Build history of the part. All positions in model axes, mm. A direction names the side the tool comes from. Coordinates: 2 decimals unless noted, no trailing zeros. Write each loop counter-clockwise with the first axis right and the second up, starting at its lowest first coordinate (ties: lowest second). Pieces come first, ordered by that corner, then holes.
```python
from build123d import *

# Parameters (mm, degrees)
SKETCH1_R          = 72.5
BASE_FLANGE1_DEPTH = 1


# Read off the part's stored shape, not the designer's step: Edge-Flange1
# Sheet-metal steps are written as plain solids
with BuildPart() as part:
    # Sketch1 → Base-Flange1 (new body)
    with BuildSketch(Plane(origin=(0, 0, 0), x_dir=(1, 0, 0), z_dir=(0, 1, 0))):
        with Locations(Location((0, 0, 0), (0, 0, 270))):
            Circle(SKETCH1_R)
    extrude(amount=-BASE_FLANGE1_DEPTH)

    # Edge-Flange1 outline → Edge-Flange1 (revolve)
    with BuildSketch(Plane.XY):
        with BuildLine():
            Line((77.5, 19), (76.5, 19))
            Line((76.5, 19), (76.5, 3))
            ThreePointArc((76.5, 3), (75.621320344, 0.878679656), (73.5, 0))
            Line((73.5, 0), (72.5, 0))
            Line((72.5, 0), (72.5, -1))
            Line((72.5, -1), (73.5, -1))
            ThreePointArc((73.5, -1), (76.328427125, 0.171572875), (77.5, 3))
            Line((77.5, 3), (77.5, 19))
        make_face()
    revolve(axis=Axis((0, 0, 0), (0, 1, 0)))


solid = part.part
```
1. Saw through at B-B on x = 0. List the corners of the cut face in (y, z).
Computed values:
outline: (-1, -73.5) arc R4 ccw to (3, -77.5) - (19, -77.5) - (19, -76.5) - (3, -76.5) arc R3 cw to (0, -73.5) - (0, 73.5) arc R3 cw to (3, 76.5) - (19, 76.5) - (19, 77.5) - (3, 77.5) arc R4 ccw to (-1, 73.5) - close
2. Flat gauge pins, fed straight in: pin 1 (8 mm diameter, centred on x = 58.5, y = 14, fed in from -Z); pin 2 (10 mm diameter, centred on y = 16.5, z = 10, fed in from +X); pin 3 (3 mm diameter, centred on x = 8, y = 12.5, fed in from +Z). Where does each tip first touch, or does it go through?
Computed values:
pin 1: stops at z = -55.1
pin 2: stops at x = 77.34
pin 3: stops at z = 77.23
3. Mould opens along X. For faces 1 (the face through (1, -1, -1)), 2 (the face through (-60.708, 10.888, 46.549)), 3 (the face through (-16.8, 11.112, 75.657)) say: +X half, -X half, draft (parallel to the pull), parting line (faces both ways), or undercut.
Computed values:
face 1: draft
face 2: undercut
face 3: parting line
4. 3-axis set-ups, long thin cutter, end or side, ignore diameter. For faces 4 (the face through (51.3, 19, 57)), 5 (the face through (-1, 0, -1)): which of +Z, -Z, +X, -X, +Y, -Y reach the whole face in a straight line?
Computed values:
face 4: +Z, -Z, +X, -X, +Y
face 5: +Y
5. Saw through at A-A on y = 9.75. List the corners of the cut face in (x, z), plus the area to 3 significant figures.
Computed values:
outline: circle Ø155 at (0, 0); hole circle Ø153 at (0, 0)
area: 484 mm2
6. Probe line 1 along Z through (x, y) = (0, 15.25); line 2 along Y through (x, z) = (-12.5, -30). List the from-to ranges inside material, lowest first.
Computed values:
line 1: z = -77.5 to -76.5, 76.5 to 77.5
line 2: y = -1 to 0
7. Saw through at C-C on z = 0. List the corners of the cut face in (x, y), plus the area to 3 significant figures.
Computed values:
outline: (-77.5, 3) arc R4 ccw to (-73.5, -1) - (73.5, -1) arc R4 ccw to (77.5, 3) - (77.5, 19) - (76.5, 19) - (76.5, 3) arc R3 cw to (73.5, 0) - (-73.5, 0) arc R3 cw to (-76.5, 3) - (-76.5, 19) - (-77.5, 19) - close
area: 190 mm2
